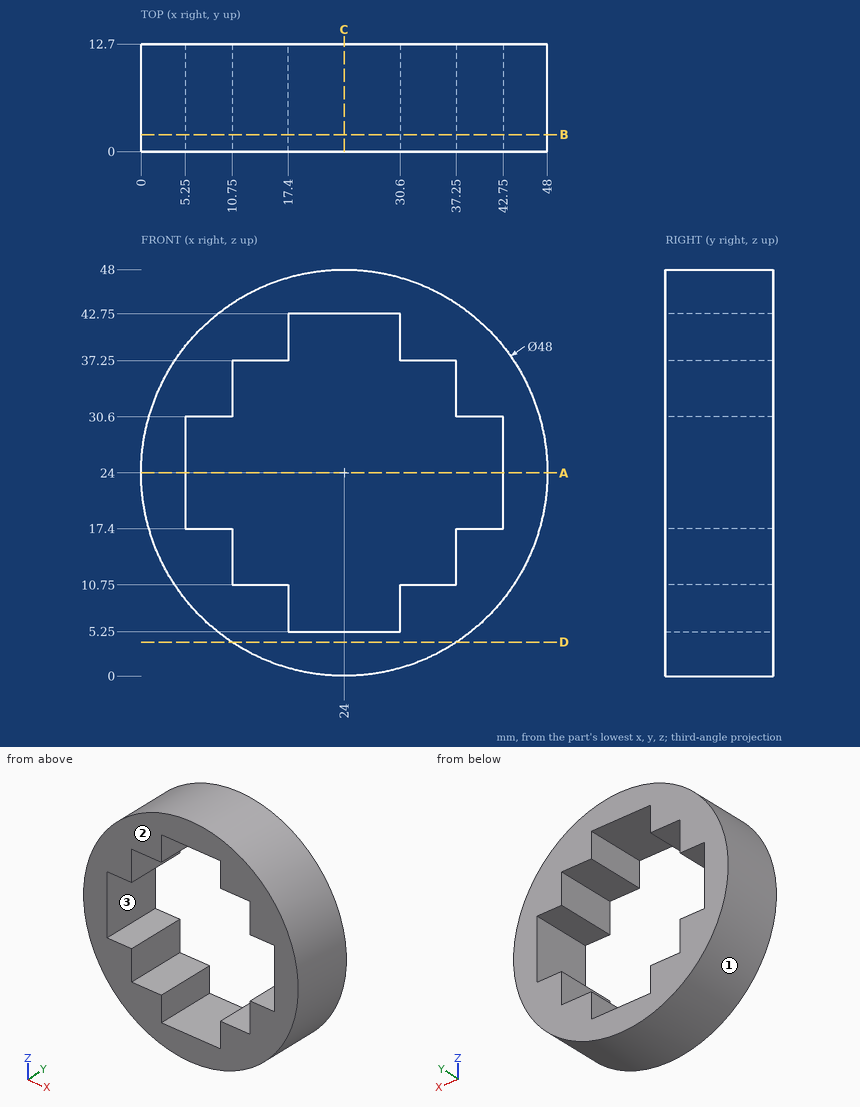
The figure shows three views and two pictorial views of one solid part (mm, origin at its lowest corner). Answer the questions. Coordinates: 2 decimals unless noted, no trailing zeros. Loops run counter-clockwise (first coordinate to the right, second up) from the corner with the lowest first, then second, coordinate; pieces in that order, holes last. Notation, with made-up numbers: (74.5, -13) - (115.5, -13) arc R25 cw to (115.5, 7) - close; hole circle Ø10 at (59, -5.75). An arc over 180 degrees is marked (long way). Use a Markdown table: item, result. Add a question column.
1) The mould has two halves that part along X. Classify the marked faces 1, 2 and 3: released by +X, released by -X, zero draft, split by the parting line, or undercut.
2) Find the intervals of material crossed by line 1 (X direction, y = 3, z = 29.5); line 2 (Z direction, x = 41, y = 7); line 3 (Z direction, x = 20, y = 3.25), in increasing order.
3) The part is cut by section A-A, the plane z = 24. Give the vertices of the cut face in (x, y), and give its area (3 significant figures).
4) Given pin 1 (3 mm diameter, centred on y = 4, z = 8.5, fed in from +X); pin 2 (5.5 mm diameter, centred on y = 9.5, z = 35, fed in from -X); pin 3 (7.5 mm diameter, centred on x = 34.5, y = 8.5, fed in from +Z); pin 4 (4 mm diameter, centred on x = 36.5, z = 14, fed in from +Y), each flat-ended and moving along its own axis, determine where each tip first touches the part or whether it passes through.
5) The part is cut by section C-C, the plane x = 24. Give the vertices of the cut face in (y, z).
6) The part is cut by section D-D, the plane z = 4. Give the vertices of the cut face in (x, y), and give its area (3 significant figures).
7) The part is cut by section B-B, the plane y = 2. Give the vertices of the cut face in (x, z), and give its area (3 significant figures).
Here are the results:
| question | item | result |
|---|---|---|
| 1 | face 1 | split by the parting line |
| 1 | face 2 | zero draft |
| 1 | face 3 | undercut |
| 2 | line 1 | x = 0.64 to 5.25, 42.75 to 47.36 |
| 2 | line 2 | z = 7.06 to 17.4, 30.6 to 40.94 |
| 2 | line 3 | z = 0.34 to 5.25, 42.75 to 47.66 |
| 3 | outline | (0, 0) - (5.25, 0) - (5.25, 12.7) - (0, 12.7) - close; (42.75, 0) - (48, 0) - (48, 12.7) - (42.75, 12.7) - close |
| 3 | area | 133 mm^2 |
| 4 | pin 1 | stops at x = 43.49 |
| 4 | pin 2 | stops at x = 1.46 |
| 4 | pin 3 | stops at z = 47.03 |
| 4 | pin 4 | stops at y = 12.7 |
| 5 | outline | (0, 0) - (12.7, 0) - (12.7, 5.25) - (0, 5.25) - close; (0, 42.75) - (12.7, 42.75) - (12.7, 48) - (0, 48) - close |
| 6 | outline | (10.73, 0) - (37.27, 0) - (37.27, 12.7) - (10.73, 12.7) - close |
| 6 | area | 337 mm^2 |
| 7 | outline | circle Ø48 at (24, 24); hole (5.25, 17.4) - (10.75, 17.4) - (10.75, 10.75) - (17.4, 10.75) - (17.4, 5.25) - (30.6, 5.25) - (30.6, 10.75) - (37.25, 10.75) - (37.25, 17.4) - (42.75, 17.4) - (42.75, 30.6) - (37.25, 30.6) - (37.25, 37.25) - (30.6, 37.25) - (30.6, 42.75) - (17.4, 42.75) - (17.4, 37.25) - (10.75, 37.25) - (10.75, 30.6) - (5.25, 30.6) - close |
| 7 | area | 817 mm^2 |
